```python
from build123d import *

# Parameters (mm, degrees)
BOSS_EXTRUDE1_DEPTH = 24
SKETCH3_W           = 10.19023154
SKETCH3_H           = 1.95
BOSS_EXTRUDE2_DEPTH = 3
SKETCH5_R           = 18
CUT_EXTRUDE1_DEPTH  = 30.921809562
CHAMFER1_SIZE       = 0.5
FILLET1_R           = 1
SKETCH6_R           = 1.275
CUT_EXTRUDE2_DEPTH  = 30.14023621
SKETCH7_R           = 1
CUT_EXTRUDE3_DEPTH  = 31.169687207
FILLET2_R           = 2


with BuildPart() as part:
    # Sketch2 → Boss-Extrude1 (new body)
    with BuildSketch(Plane.XY):
        Polygon((-14.57097685, 4.125), (-4.07097685, 4.125), (-4.07097685, 0), (0, 0), (0.02932299, 2.4), (-8.612483466, 7.8), (-14.57097685, 7.8), align=None)
    extrude(amount=BOSS_EXTRUDE1_DEPTH)

    # Sketch3 → Boss-Extrude2 (add)
    with BuildSketch(Plane(origin=(1.086787174, 1.739223041, 0), x_dir=(0.8480480961564272, -0.5299192642332031, 0), z_dir=(0.5299192642332031, 0.8480480961564273, 0))):
        with Locations((-6.342054698, -0.975)):
            Rectangle(SKETCH3_W, SKETCH3_H)
        with Locations((-6.342054698, -23.025)):
            Rectangle(SKETCH3_W, SKETCH3_H)
    extrude(amount=BOSS_EXTRUDE2_DEPTH)

    # Sketch5 → Cut-Extrude1 (cut, through all)
    with BuildSketch(Plane(origin=(0, 0, 0), x_dir=(0, 0, -1), z_dir=(0.9999253696604522, -0.012217000835240004, 0))):
        with Locations((-8.95, -16.33799405)):
            Circle(SKETCH5_R)
    extrude(amount=-CUT_EXTRUDE1_DEPTH, mode=Mode.SUBTRACT)

    # Chamfer1
    chamfer1_edges = [part.edges().sort_by_distance(p)[0] for p in [
        (-2.701822445, 7.644144288, 0),
        (-2.701822445, 7.644144288, 24),
    ]]
    chamfer(chamfer1_edges, length=CHAMFER1_SIZE)

    # Fillet1
    fillet1_edges = [part.edges().sort_by_distance(p)[0] for p in [
        (-14.57097685, 5.9625, 24),
        (-14.57097685, 5.9625, 0),
    ]]
    fillet(fillet1_edges, radius=FILLET1_R)

    # Sketch6 → Cut-Extrude2 (cut, through all)
    with BuildSketch(Plane(origin=(0, 7.8, 0), x_dir=(1, 0, 0), z_dir=(0, 1, 0))):
        with Locations(Location((-11.22097685, -17.05, 0), (0, 0, 180))):
            Circle(SKETCH6_R)
        with Locations(Location((-11.22097685, -7.55, 0), (0, 0, 180))):
            Circle(SKETCH6_R)
    extrude(amount=-CUT_EXTRUDE2_DEPTH, mode=Mode.SUBTRACT)

    # Sketch7 → Cut-Extrude3 (cut, through all)
    with BuildSketch(Plane(origin=(2.676544967, 4.283367329, 0), x_dir=(0.8480480961564271, -0.5299192642332031, 0), z_dir=(0.5299192642332031, 0.8480480961564271, 0))):
        with Locations((-9.151078225, -17.05)):
            Circle(SKETCH7_R)
        with Locations((-9.151078225, -7.55)):
            Circle(SKETCH7_R)
    extrude(amount=-CUT_EXTRUDE3_DEPTH, mode=Mode.SUBTRACT)

    # Fillet2
    fillet2_edges = [part.edges().sort_by_distance(p)[0] for p in [
        (-8.612483466, 7.8, 23.025),
        (-8.612483466, 7.8, 0.975),
    ]]
    fillet(fillet2_edges, radius=FILLET2_R)


solid = part.part
```
Work out the finished part from the listing and answer in its coordinate system (mm). A direction names the side the tool comes from. Give positions to 0.01 mm unless a question says otherwise; leave off trailing zeros. Loops run counter-clockwise (first coordinate to the right, second up) from the corner with the lowest first, then second, coordinate; pieces in that order, holes last. Notation, with made-up numbers: (61.25, 12.5) - (102.25, 12.5) arc R27 cw to (102.25, 37.5) - close; hole circle Ø8 at (41.5, -7.75). An arc over 180 degrees is marked (long way). One line per question, with ' | ' between items.
(1) The part is cut by section C-C (y = 8.25). Write down the section's boundary in (x, z), then the cut area to 3 significant figures.
Recorded:
outline: (-8.46, 0) - (-4.61, 0) - (-3.67, 0.5) - (-3.67, 1.95) - (-8.46, 1.95) - close; (-8.46, 22.05) - (-3.67, 22.05) - (-3.67, 23.5) - (-4.61, 24) - (-8.46, 24) - close | area: 18.2 mm²
(2) The part is cut by section D-D (z = 3.25). Write down the section's boundary in (x, y) (3 decimals).
Recorded:
outline: (-14.571, 4.125) - (-4.071, 4.125) - (-4.071, 0.785) - (0.009, 0.736) - (0.029, 2.4) - (-8.612, 7.8) - (-14.571, 7.8) - close
(3) Straight lines are drawn through the part: probe 1 along Z at (x, y) = (-3.75, 5.5); probe 2 along Z at (x, y) = (-7.5, 4.5); probe 3 along Y at (x, z) = (-12.25, 14.25) (3 decimals). For each, find the intervals that lie inside material, in ascending order.
Recorded:
probe 1: z = 0 to 1.95, 22.05 to 24 | probe 2: z = 0 to 6.64, 8.46 to 16.14, 17.96 to 24 | probe 3: y = 4.125 to 7.8
(4) The mould has two halves that part along Z. Classify faces 1 (the face through (-2.89, 7.47, 0.25)), 2 (the face through (-14.571, 6, 12)), 3 (the face through (-12, 7.8, 12)): +Z half, -Z half, draft (parallel to the pull), parting line (faces both ways), or undercut.
Recorded:
face 1: -Z half | face 2: draft | face 3: undercut
(5) Each of these flat-tipped pins is pushed along its axis until it touches: pin 1 Ø1.8 at (x, z) = (-12, 8) entering from +Y; pin 2 Ø3 at (y, z) = (2.5, 12) entering from -X. Where does it stop, or does it pass through?
Recorded:
pin 1: stops at y = 7.8 | pin 2: stops at x = -4.07
(6) The part is cut by section A-A (z = 7.55). Write down the section's boundary in (x, y) (3 decimals), then the cut area to 3 significant figures.
Recorded:
outline: (-14.571, 4.125) - (-12.496, 4.125) - (-12.496, 7.8) - (-14.571, 7.8) - close; (-9.946, 4.125) - (-9.392, 4.125) - (-7.522, 7.118) - (-8.612, 7.8) - (-9.946, 7.8) - close; (-7.034, 4.125) - (-4.071, 4.125) - (-4.071, 1.657) - (0.02, 1.607) - (0.029, 2.4) - (-5.826, 6.059) - close | area: 25.4 mm²
(7) A tool of negligible diameter and unlimited length cuts with its end or side. For faces 4 (the face through (-4.23, 5.06, 11.86)), 5 (the face through (-4.071, 3, 12)), 6 (the face through (0.81, 3.65, 0.99)), from which of +Z, -Z, +X, -X, +Y, -Y can it reach the whole face along a straight path? Write none if from no direction.
Recorded:
face 4: +X, +Y | face 5: +Z, -Z, -X, -Y | face 6: +Z, -Z, +X, -Y
(8) The part is cut by section B-B (x = -12). Write down the section's boundary in (y, z) (3 decimals).
Recorded:
outline: (4.125, 0) - (7.8, 0) - (7.8, 6.541) - (4.125, 6.541) - close; (4.125, 8.559) - (7.8, 8.559) - (7.8, 16.041) - (4.125, 16.041) - close; (4.125, 18.059) - (7.8, 18.059) - (7.8, 24) - (4.125, 24) - close
